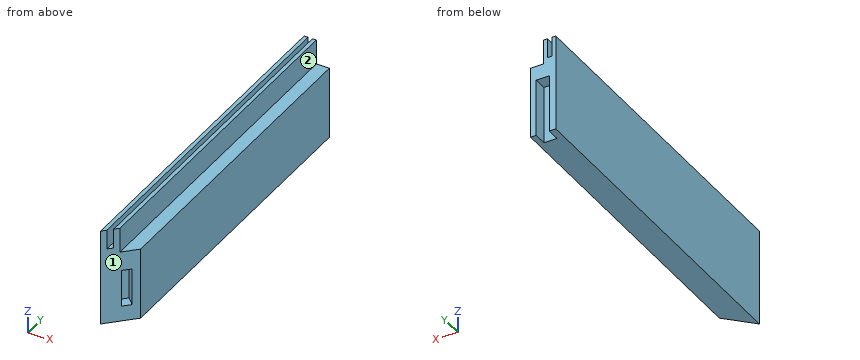
from build123d import *

# Parameters (mm, degrees)
BOSS_EXTRUDE1_DEPTH = 265.3
SKETCH2_W           = 10
SKETCH2_H           = 44
CUT_EXTRUDE1_DEPTH  = 10
SKETCH3_W           = 271.149403365
SKETCH3_H           = 159.03985052
CUT_EXTRUDE2_DEPTH  = 31
SKETCH4_W           = 28
SKETCH4_H           = 7
CUT_EXTRUDE3_DEPTH  = 8
SKETCH5_W           = 28.4
SKETCH5_H           = 7.4
CUT_EXTRUDE4_DEPTH  = 8


with BuildPart() as part:
    # Sketch1 → Boss-Extrude1 (new body)
    with BuildSketch(Plane(origin=(0, 0, 0), x_dir=(1, 0, 0), z_dir=(0, 1, 0))):
        Polygon((-51.505795374, 37), (-32.205795374, 37), (-32.205795374, -18), (-42.205795374, -18), (-42.205795374, -37), (-45.205795374, -37), (-45.205795374, -22), (-48.505795374, -22), (-48.505795374, -37), (-51.505795374, -37), align=None)
    extrude(amount=BOSS_EXTRUDE1_DEPTH)

    # Sketch2 → Cut-Extrude1 (cut)
    with BuildSketch(Plane(origin=(0, 265.3, 0), x_dir=(1, 0, 0), z_dir=(0, 1, 0))):
        with Locations((-41.505795374, 15)):
            Rectangle(SKETCH2_W, SKETCH2_H)
    extrude(amount=-CUT_EXTRUDE1_DEPTH, mode=Mode.SUBTRACT)

    # Sketch3 → Cut-Extrude2 (cut)
    with BuildSketch(Plane(origin=(-25.752897687, 25.752897687, 0), x_dir=(0, 0, 1), z_dir=(0.7071067811865488, -0.7071067811865464, 0))):
        with Locations((3.075588753, 19.523863597)):
            Rectangle(SKETCH3_W, SKETCH3_H)
    extrude(amount=CUT_EXTRUDE2_DEPTH, mode=Mode.SUBTRACT)

    # Sketch4 → Cut-Extrude3 (cut)
    with BuildSketch(Plane(origin=(-25.752897687, 25.752897687, 0), x_dir=(0, 0, -1), z_dir=(0.7071067811865487, -0.7071067811865465, 0))):
        with Locations((11, -18.625775426)):
            Rectangle(SKETCH4_W, SKETCH4_H)
    extrude(amount=-CUT_EXTRUDE3_DEPTH, mode=Mode.SUBTRACT)

    # Sketch5 → Cut-Extrude4 (cut)
    with BuildSketch(Plane(origin=(-25.752897687, 25.752897687, 0), x_dir=(0, 0, -1), z_dir=(0.7071067811865487, -0.7071067811865465, 0))):
        with Locations((11, -18.625775426)):
            Rectangle(SKETCH5_W, SKETCH5_H)
    extrude(amount=-CUT_EXTRUDE4_DEPTH, mode=Mode.SUBTRACT)


solid = part.part
Source: CAD feature listing. Evaluate the final solid. Frame: model axes, mm. Face numbers are marked on the shaded views. A direction names the side the tool comes from. Coordinates: 2 decimals unless noted, no trailing zeros. Order: outer loops, then holes, each group sorted by start corner. A loop starts at its lowest first (then second) coordinate and runs counter-clockwise, first axis right, second up. Notation, with made-up numbers: M -30.5,48 L -26.5,48 A19 ccw -26.5,73 Z; hole C 66.25,-1.75 d6. An arc over 180 degrees is marked long. Write each question's results on one line, items separated by ' | '. Start each with the question number.
Item 1: Cut plane A-A (z = -27.5). Return loops of the section in (x, y).
Item 2: Cut plane D-D (z = 12). Return loops of the section in (x, y).
Item 3: Line query: probe 1 along X at (y, z) = (13, 26.5); probe 2 along Z at (x, y) = (-39.25, 253); probe 3 along Z at (x, y) = (-45.75, 218). Output: solid intervals per line, ascending.
Item 4: Cut plane B-B (y = 107.5). Return loops of the section in (x, z), and give its area (3 significant figures).
Item 5: Cut plane C-C (z = -12). Return loops of the section in (x, y).
Item 6: Set-up query: the marked faces 1 and 2. Return all of +Z, -Z, +X, -X, +Y, -Y with unobstructed straight access to the full face (end or side cutting, diameter ignored); none if empty.
Item 7: First-contact query: pin 1 Ø5 at (x, y) = (-43, 259.5) entering from -Z; pin 2 Ø10 at (x, z) = (-37, -16.5) entering from -Y; pin 3 Ø5.5 at (y, z) = (110.5, 25) entering from +X. Flat tips, straight axial feed; report the tip coordinate or a pass-through.
Checked values:
1) outline: M -51.51,0 L -32.21,19.3 L -32.21,265.3 L -36.51,265.3 L -36.51,255.3 L -46.51,255.3 L -46.51,265.3 L -51.51,265.3 Z
2) outline: M -51.51,0 L -32.21,19.3 L -32.21,265.3 L -51.51,265.3 Z
3) probe 1: x = -51.51 to -48.51, -45.21 to -42.21 | probe 2: z = -37 to 18 | probe 3: z = -37 to 22
4) outline: M -51.51,-37 L -32.21,-37 L -32.21,18 L -42.21,18 L -42.21,37 L -45.21,37 L -45.21,22 L -48.51,22 L -48.51,37 L -51.51,37 Z | area: 1,190 mm2
5) outline: M -51.51,0 L -41.54,9.97 L -47.2,15.62 L -41.96,20.86 L -36.31,15.2 L -32.21,19.3 L -32.21,265.3 L -36.51,265.3 L -36.51,255.3 L -46.51,255.3 L -46.51,265.3 L -51.51,265.3 Z
6) face 1: +Z, -Z, +X, -Y | face 2: +Z, +X, +Y, -Y
7) pin 1: stops at z = 7 | pin 2: stops at y = 9.51 | pin 3: stops at x = -42.21
